```python
from build123d import *

# Parameters (mm, degrees)
SKETCH004_R      = 1.5
EXTRUDE004_DEPTH = 2
BOX002_W         = 20
BOX002_H         = 43.25
BOX002_DEPTH     = 1.6


with BuildPart() as holesextrude:
    # Sketch004 (on Face6 of Box002) → Extrude004 (new body)
    with BuildSketch(Plane(origin=(11, 0, 1.6), x_dir=(0, -1, 0), z_dir=(0, 0, 1))):
        with Locations((11.4, 38.171532)):
            Circle(SKETCH004_R)
        with Locations((11.4, 8.471532)):
            Circle(SKETCH004_R)
    extrude(amount=-EXTRUDE004_DEPTH)


with BuildPart() as board002:
    # Box002 → Box002 (new body)
    with BuildSketch(Plane(origin=(11, 0, 0), x_dir=(0, -1, 0), z_dir=(0, 0, 1))):
        with Locations((10, 21.625)):
            Rectangle(BOX002_W, BOX002_H)
    extrude(amount=BOX002_DEPTH)

    # Cut001: cut HolesExtrude
    add(holesextrude.part, mode=Mode.SUBTRACT)


solid = board002.part
```
Model file for the job. Use its own axes, mm. Coordinates: 2 decimals unless noted, no trailing zeros. Loops run counter-clockwise (first coordinate to the right, second up) from the corner with the lowest first, then second, coordinate; pieces in that order, holes last. Notation, with made-up numbers: M 0,-1.75 L 8,-1.75 A24 cw 8,14.25 Z; hole C 73.25,-38 d5. An arc over 180 degrees is marked long. Use CSV: the item, a comma, the result in double quotes. Start each with the question number.
1. Band-saw the part on C-C, the plane z = 0.8. List the corners of the cut face in (x, y).
2. Flat gauge pin, fed straight in: pin 1 (1.5 mm diameter, centred on x = 45, y = -2.5, fed in from -Z). Where does the tip first touch, or does it go through?
3. Band-saw the part on A-A, the plane y = -11.4. List the corners of the cut face in (x, z).
4. Probe probe 1 along X at (y, z) = (-11.4, 1.2); probe 2 along X at (y, z) = (-11.75, 0.35); probe 3 along Y at (x, z) = (49.5, 0.2). List the from-to ranges inside material, lowest first. Write a range as [from, to].
5. Two-plate mould, pull along Y, no slides. Class faces 1 (the flat face through (32, -20, 1)), 2 (the cylindrical face through (48.26, -10.21, 0.81)), 3 (the flat face through (33, -10, 0)): pulls with the +Y half, pulls with the -Y half, needs draft (parallel to the pull), parting line crosses it, or undercut.
6. Band-saw the part on B-B, the plane x = 20. List the corners of the cut face in (y, z).
Entries:
1,outline,"M 11,-20 L 54.25,-20 L 54.25,0 L 11,0 Z; hole C 19.47,-11.4 d3; hole C 49.17,-11.4 d3"
2,pin 1,"stops at z = 0"
3,outline,"M 11,0 L 17.97,0 L 17.97,1.6 L 11,1.6 Z; M 20.97,0 L 47.67,0 L 47.67,1.6 L 20.97,1.6 Z; M 50.67,0 L 54.25,0 L 54.25,1.6 L 50.67,1.6 Z"
4,probe 1,"x = [11, 17.97], [20.97, 47.67], [50.67, 54.25]"
4,probe 2,"x = [11, 18.01], [20.93, 47.71], [50.63, 54.25]"
4,probe 3,"y = [-20, -12.86], [-9.94, 0]"
5,face 1,"pulls with the -Y half"
5,face 2,"undercut"
5,face 3,"needs draft"
6,outline,"M -20,0 L -12.8,0 L -12.8,1.6 L -20,1.6 Z; M -10,0 L 0,0 L 0,1.6 L -10,1.6 Z"
